CAD build for the part. Positions are in the model's coordinates, mm. Face numbers are marked on the shaded views. Coordinates: 2 decimals unless noted, no trailing zeros. Loops run counter-clockwise (first coordinate to the right, second up) from the corner with the lowest first, then second, coordinate; pieces in that order, holes last.
1) Wall check: line 1 along Y through (x, z) = (0, 2.05); line 2 along Y through (x, z) = (0, 0.25); line 3 along Z through (x, y) = (-0.8, -1.85). Give the ranges that are in metal, low to high.
2) Saw through at C-C, the plane z = 2.95. Write the cut outline in (x, y).
3) Two-plate mould, pull along X, no slides. Class the marked faces 1, 2 and 3: +X half, -X half, draft (parallel to the pull), parting line (faces both ways), or undercut.
4) Saw through at D-D, the plane y = 2. Write the cut outline in (x, z).
5) Pin check, flat tip, straight feed: pin 1 Ø1.5 at (x, z) = (-2, 1.5) entering from +Y. Stop position of the tip, or through.
6) Saw through at A-A, the plane y = 0. Write the cut outline in (x, z), and give its area (3 significant figures).
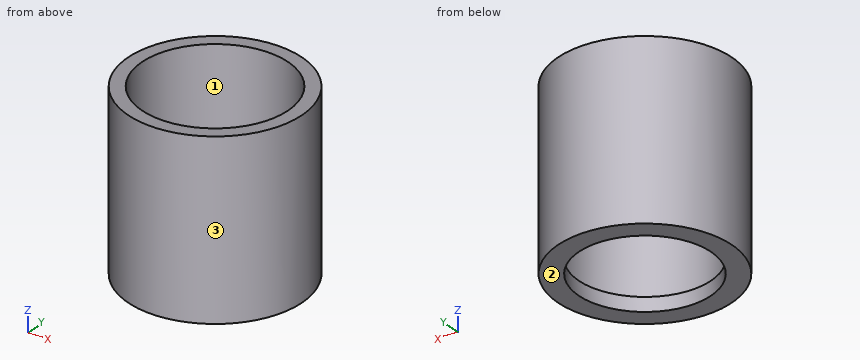
```python
from build123d import *

# Parameters (mm, degrees)
F0_R     = 2.5
F1_DEPTH = 5
F2_T     = -0.4
F3_R     = 1.9
F4_DEPTH = 25


with BuildPart() as f1:
    # F0 (on Top) → F1 (new body)
    with BuildSketch(Plane.XY):
        Circle(F0_R)
    extrude(amount=F1_DEPTH)

    # F2
    f2_openings = [f1.faces().sort_by_distance(p)[0] for p in [
        (0, 0, 5),
    ]]
    offset(amount=F2_T, openings=f2_openings)

    # F3 (on face) → F4 (cut)
    with BuildSketch(Plane(origin=(0, 0, 0), x_dir=(1, 0, 0), z_dir=(0, 0, -1))):
        Circle(F3_R)
    extrude(amount=-F4_DEPTH, mode=Mode.SUBTRACT)


solid = f1.part
```
Data:
1. line 1: y = -2.5 to -2.1, 2.1 to 2.5
1. line 2: y = -2.5 to -1.9, 1.9 to 2.5
1. line 3: z = 0 to 0.4
2. outline: circle Ø5 at (0, 0); hole circle Ø4.2 at (0, 0)
3. face 1: undercut
3. face 2: draft
3. face 3: parting line
4. outline: (-1.5, 0) - (1.5, 0) - (1.5, 5) - (0.64, 5) - (0.64, 0.4) - (-0.64, 0.4) - (-0.64, 5) - (-1.5, 5) - close
5. pin 1: stops at y = 2.17
6. outline: (-2.5, 0) - (-1.9, 0) - (-1.9, 0.4) - (-2.1, 0.4) - (-2.1, 5) - (-2.5, 5) - close; (1.9, 0) - (2.5, 0) - (2.5, 5) - (2.1, 5) - (2.1, 0.4) - (1.9, 0.4) - close
6. area: 4.16 mm2
